Design review of the part built by this model. Coordinates are the model's own, in mm. Coordinates: 2 decimals unless noted, no trailing zeros. Loops run counter-clockwise (first coordinate to the right, second up) from the corner with the lowest first, then second, coordinate; pieces in that order, holes last. Notation, with made-up numbers: M 69.5,-2 L 88.5,-2 A24 ccw 88.5,21 Z; hole C 74,17 d1. An arc over 180 degrees is marked long. One line per item, written item: value.
```python
from build123d import *

# Parameters (mm, degrees)
F0_W     = 28.0245169997
F0_H     = 34.0497903526
F1_DEPTH = 39.53846
F2_SIZE2 = 5.08
F2_SIZE  = 4.2626261264


with BuildPart() as f1:
    # F0 (on Top) → F1 (new body)
    with BuildSketch(Plane.XY):
        with Locations((14.0122584999, 17.0248951763)):
            Rectangle(F0_W, F0_H)
    extrude(amount=F1_DEPTH)

    # F2
    f2_edges = [f1.edges().sort_by_distance(p)[0] for p in [
        (28.024517, 34.04979, 19.76923),
        (28.024517, 17.024895, 39.53846),
    ]]
    f2_side = f1.faces().sort_by_distance((28.024517, 17.024895, 19.76923))[0]
    chamfer(f2_edges, length=F2_SIZE, length2=F2_SIZE2, reference=f2_side)


solid = f1.part
```
(1) We need section A-A on z = 36.5. State the section outline as (x, y) points.
Reply:
outline: M 0,0 L 26.57,0 L 26.57,31.01 L 22.94,34.05 L 0,34.05 Z
(2) To check wall thickness, follow line 1 along Z through (x, y) = (23.25, 23); line 2 along Z through (x, y) = (25, 11); line 3 along X through (y, z) = (21.5, 37). State the ranges of each line that lie inside material, in increasing order. Write a range as [from, to].
Reply:
line 1: z = [0, 39.28]
line 2: z = [0, 37.81]
line 3: x = [0, 25.97]
(3) We need section B-B on x = 26.25. State the section outline as (y, z) points, then the cut area to 3 significant figures.
Reply:
outline: M 0,0 L 31.28,0 L 31.28,36.76 L 0,36.76 Z
area: 1,150 mm2
